Autodesk Inventor part; units mm, degrees
ref_plane "YZ Plane" through (0, 0, 0) normal (1, 0, 0) x (0, 1, 0)
ref_plane "XZ Plane" through (0, 0, 0) normal (0, 1, 0) x (-1, 0, 0)
ref_plane "XY Plane" through (0, 0, 0) normal (0, 0, 1) x (1, 0, 0)
sketch "Эскиз4" plane through (0, 0, 0) normal (0, 0, 1) x (1, 0, 0)
  line L0 (45.2395, 25.2453) -> (-44.981, 25.2453)
  line L1 (-44.981, 25.2453) -> (-44.981, -24.4084)
  line L2 (-44.981, -24.4084) -> (45.2395, -24.4084)
  line L3 (45.2395, -24.4084) -> (45.2395, 25.2453)
  point P0 (0, 0)
extrude "Прямоугольник_" add sketch "Эскиз4" along normal blind 15
sketch "Прямоугольник" plane through (0, 0, 0) normal (0, 0, 1) x (1, 0, 0)
  line L0 (-77.4921, 158.0418) -> (133.4103, 158.0418) construction
  line L1 (133.4103, 158.0418) -> (133.4103, -71.9132) construction
  line L2 (133.4103, -71.9132) -> (-77.4921, -71.9132) construction
  line L3 (-77.4921, -71.9132) -> (-77.4921, 158.0418) construction
  line L4 (44.9907, 25.2614) -> (-45.0093, 25.2614)
  line L5 (-45.0093, 25.2614) -> (-45.0093, -24.7386)
  line L6 (-45.0093, -24.7386) -> (44.9907, -24.7386)
  line L7 (44.9907, -24.7386) -> (44.9907, 25.2614)
  point P0 (0, 0)
  dimension "d17" = 90
  dimension "d20" = 50
sketch "Три отверстия по краям" plane through (0, 0, 15) normal (0, 0, 1) x (1, 0, 0)
  circle A0 centre (-34.9124, 0) radius 5
  circle A1 centre (35.035, 15.2594) radius 5
  circle A2 centre (35.035, -14.8643) radius 5
  point P0 (0, 0)
  dimension "d12" = 10
  dimension "d13" = 10
  dimension "d14" = 10
extrude "3 отверстия по краям" cut sketch "Три отверстия по краям" against normal blind 800
sketch "Возвышенность по центру" plane through (0, 0, 15) normal (0, 0, 1) x (1, 0, 0)
  circle A0 centre (0, 0) radius 15
  dimension "d21" = 30
extrude "Возвышенность" add sketch "Возвышенность по центру" along normal blind 25
sketch "Эскиз7" plane through (0, 0, 0) normal (0, 0, -1) x (-1, 0, 0)
  circle A0 centre (0, 0) radius 9
  dimension "d24" = 18
extrude "Внутренняя часть внутри возв" cut sketch "Эскиз7" against normal blind 38
properties part number "Основание БЕЗ опор по бокам"
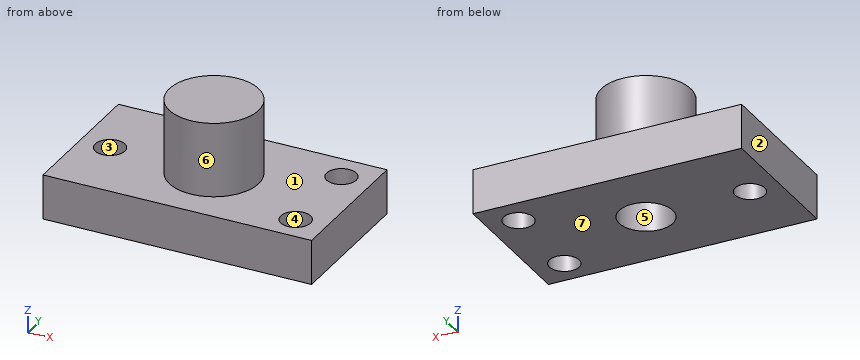
The listing builds one solid part. Answer for the finished solid, in the listing's coordinates (mm). Face numbers are marked on the shaded views. A direction names the side the tool comes from. Coordinates: 2 decimals unless noted, no trailing zeros. Write each loop counter-clockwise with the first axis right and the second up, starting at its lowest first coordinate (ties: lowest second). Pieces come first, ordered by that corner, then holes.
Q1. Given P1, Ø20, axis at x = 4, y = 4, coming from the -Z side; P2, Ø4, axis at x = -22, y = 9.5, coming from the +Z side; P3, Ø8, axis at y = -10.5, z = 33, coming from the +X side; P4, Ø10, axis at y = -7, z = 29.5, coming from the +X side, each flat-ended and moving along its own axis, determine where each tip first touches the part or whether it passes through.
Returned:
P1: stops at z = 0
P2: stops at z = 15
P3: stops at x = 13.52
P4: stops at x = 14.87
Q2. The mould has two halves that part along X. Classify the marked faces 1, 2, 3 and 4: released by +X, released by -X, zero draft, split by the parting line, or undercut.
Returned:
face 1: zero draft
face 2: released by -X
face 3: undercut
face 4: undercut
Q3. Section D-D, the plane x = 34 is taken. Write down the section's boundary in (y, z).
Returned:
outline: (-24.41, 0) - (-19.76, 0) - (-19.76, 15) - (-24.41, 15) - close; (-9.97, 0) - (10.37, 0) - (10.37, 15) - (-9.97, 15) - close; (20.15, 0) - (25.25, 0) - (25.25, 15) - (20.15, 15) - close
Q4. Which of the six approach directions +Z, -Z, +X, -X, +Y, -Y give full straight-line access (tool end or side, diameter ignored) to the marked faces 5, 6 and 7?
Returned:
face 5: -Z
face 6: +Z
face 7: -Z, +X, -X, +Y, -Y
Q5. Section C-C, the plane z = 14 is taken. Write down the section's boundary in (x, y) (1 decimal).
Returned:
outline: (-45, -24.4) - (45.2, -24.4) - (45.2, 25.2) - (-45, 25.2) - close; hole circle Ø10 at (-34.9, 0); hole circle Ø18 at (0, 0); hole circle Ø10 at (35, -14.9); hole circle Ø10 at (35, 15.3)
Q6. Section B-B, the plane x = -31 is taken. Write down the section's boundary in (y, z).
Returned:
outline: (-24.41, 0) - (-3.11, 0) - (-3.11, 15) - (-24.41, 15) - close; (3.11, 0) - (25.25, 0) - (25.25, 15) - (3.11, 15) - close
Q7. Section A-A, the plane y = 0 is taken. Write down the section's boundary in (x, z).
Returned:
outline: (-44.98, 0) - (-39.91, 0) - (-39.91, 15) - (-44.98, 15) - close; (-29.91, 0) - (-9, 0) - (-9, 38) - (9, 38) - (9, 0) - (45.24, 0) - (45.24, 15) - (15, 15) - (15, 40) - (-15, 40) - (-15, 15) - (-29.91, 15) - close
Q8. Find the intervals of material crossed by line 1 along X through (y, z) = (15.5, 12); line 2 along Y through (x, z) = (0, 29); line 3 along Z through (x, y) = (-37.5, -20.5), in increasing order.
Returned:
line 1: x = -44.98 to 30.04, 40.03 to 45.24
line 2: y = -15 to -9, 9 to 15
line 3: z = 0 to 15
